Verification items for the finished model (mm, model axes). Face numbers are marked on the shaded views. A direction names the side the tool comes from. Give positions to 0.01 mm unless a question says otherwise; leave off trailing zeros. Order: outer loops, then holes, each group sorted by start corner. A loop starts at its lowest first (then second) coordinate and runs counter-clockwise, first axis right, second up.
from build123d import *

# Parameters (mm, degrees)
CUT_EXTRUDE1_DEPTH      = 32.654993342
CUT_EXTRUDE1_DEPTH_BACK = 32.654993342
SKETCH3_R               = 2.5


with BuildPart() as part:
    # Sketch2 → Revolve1 (revolve)
    with BuildSketch(Plane.XY, mode=Mode.PRIVATE) as revolve1_sk:
        with BuildLine():
            Line((-17.847985654, 8.103335303), (-17.847985654, -12.896664697))
            Line((-17.847985654, -12.896664697), (-13, -12.896664697))
            Line((-13, -12.896664697), (-13, -2.896664697))
            Line((-13, -2.896664697), (-10, -2.896664697))
            Line((-10, -2.896664697), (-10, 11.103335303))
            Line((-10, 11.103335303), (0, 11.103335303))
            Line((0, 11.103335303), (0, 19.103335303))
            ThreePointArc((0, 19.103335303), (-1.743114855, 19.027229265), (-3.472963553, 18.799490363))
            Line((-3.472963553, 18.799490363), (-17.847985654, 16.264786119))
            Line((-17.847985654, 16.264786119), (-17.847985654, 14.103335303))
            Line((-17.847985654, 14.103335303), (-14.5, 14.103335303))
            Line((-14.5, 14.103335303), (-14.5, 12.603335303))
            Line((-14.5, 12.603335303), (-17.847985654, 12.603335303))
            Line((-17.847985654, 12.603335303), (-17.847985654, 9.603335303))
            Line((-17.847985654, 9.603335303), (-14.5, 9.603335303))
            Line((-14.5, 9.603335303), (-14.5, 8.103335303))
            Line((-14.5, 8.103335303), (-17.847985654, 8.103335303))
        make_face()
    revolve(revolve1_sk.sketch.rotate(Axis((0, 24.760398889, 0), (0, -1, 0)), 270), axis=Axis((0, 24.760398889, 0), (0, -1, 0)))

    # Sketch3 → Cut-Extrude1 (cut, two sides: drawn at the far end of the back side and taken through both)
    with BuildSketch(Plane(origin=(0, 0, 0), x_dir=(0, 0, -1), z_dir=(1, 0, 0)).offset(-CUT_EXTRUDE1_DEPTH_BACK)):
        with Locations((0, 3.103335303)):
            Circle(SKETCH3_R)
    extrude(amount=CUT_EXTRUDE1_DEPTH + CUT_EXTRUDE1_DEPTH_BACK, mode=Mode.SUBTRACT)


solid = part.part
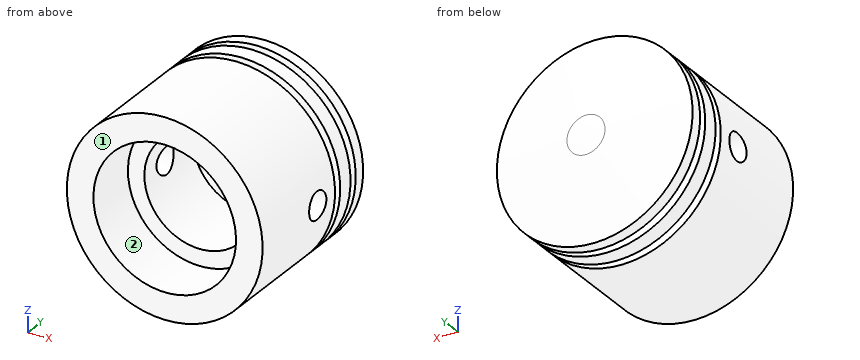
(1) Scan lines: line 1 (X direction, y = -7.25, z = 0); line 2 (Y direction, x = -13.5, z = 7); line 3 (X direction, y = 8, z = 0). Record each from-to range of solid material in increasing order.
Solved:
line 1: x = -17.85 to -13, 13 to 17.85
line 2: y = -12.9 to 8.1, 9.6 to 12.6, 14.1 to 16.73
line 3: x = -17.85 to -10, 10 to 17.85
(2) Set-up check for the marked faces 1 and 2: record each of +Z, -Z, +X, -X, +Y, -Y from which the full face is reachable in a straight line by a thin tool's end or side.
Solved:
face 1: +Z, -Z, +X, -X, -Y
face 2: -Y
(3) Section check D-D, the plane y = -8.5. Enter the section's corners in (x, z).
Solved:
outline: circle Ø35.7 at (0, 0); hole circle Ø26 at (0, 0)
(4) Go/stop test with flat-tipped pins: pin 1 (10.5 mm diameter, centred on x = -4, z = -0.5, fed in from -Y); pin 2 (10 mm diameter, centred on x = 8, z = 1.5, fed in from +Y); pin 3 (4 mm diameter, centred on y = 10.5, z = 5.5, fed in from +X); pin 4 (18 mm diameter, centred on x = 4, z = 5, fed in from +Y). Record where each tip stops, or that it passes through.
Solved:
pin 1: stops at y = 11.1
pin 2: stops at y = 18.86
pin 3: stops at x = 17.5
pin 4: stops at y = 19.1
(5) Section check C-C, the plane z = 0. Give the number of separate pieces and of enclosed holes in the cut face, then the cut area to 3 significant figures.
Solved:
separate pieces: 3
enclosed holes: 0
area: 458 mm2
